Source: CAD feature listing. Evaluate the final solid. Frame: model axes, mm. Face numbers are marked on the shaded views. A direction names the side the tool comes from. Give positions to 0.01 mm unless a question says otherwise; leave off trailing zeros. Write each loop counter-clockwise with the first axis right and the second up, starting at its lowest first coordinate (ties: lowest second). Pieces come first, ordered by that corner, then holes. Notation, with made-up numbers: (27, 42) -> (46, 42) arc R21 cw to (46, 51) -> close; hole circle Ø4 at (63.25, 42.5). An arc over 180 degrees is marked (long way). Write item = value, one per line.
from build123d import *

# Parameters (mm, degrees)
SKETCH3_W           = 14.2875
SKETCH3_H           = 19.05
BOSS_EXTRUDE1_DEPTH = 22.225
SKETCH4_W           = 9.525
SKETCH4_H           = 7.9375
BOSS_EXTRUDE2_DEPTH = 6.35
SKETCH5_W           = 6.35
SKETCH5_H           = 19.05
CUT_EXTRUDE1_DEPTH  = 16.51


with BuildPart() as part:
    # Sketch3 → Boss-Extrude1 (new body)
    with BuildSketch(Plane(origin=(0, 0, 0), x_dir=(1, 0, 0), z_dir=(0, 1, 0))):
        Rectangle(SKETCH3_W, SKETCH3_H)
    extrude(amount=BOSS_EXTRUDE1_DEPTH)

    # Sketch4 → Boss-Extrude2 (add)
    with BuildSketch(Plane(origin=(0, 22.225, 0), x_dir=(1, 0, 0), z_dir=(0, 1, 0))):
        with Locations((0, 3.96875)):
            Rectangle(SKETCH4_W, SKETCH4_H)
    extrude(amount=BOSS_EXTRUDE2_DEPTH)

    # Sketch5 → Cut-Extrude1 (cut)
    with BuildSketch(Plane.XZ):
        Rectangle(SKETCH5_W, SKETCH5_H)
    extrude(amount=-CUT_EXTRUDE1_DEPTH, mode=Mode.SUBTRACT)


solid = part.part
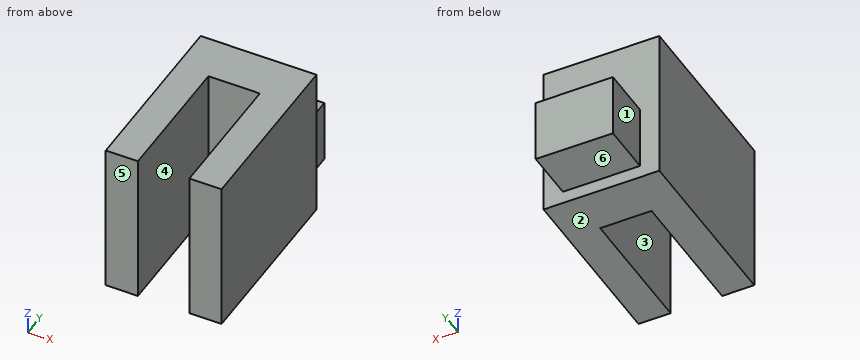
(1) Section query C-C (z = 8.25). Return loops of the section in (x, y) (3 decimals), plus the area to 3 significant figures.
Values follow:
outline = (-7.144, 0) -> (-3.175, 0) -> (-3.175, 16.51) -> (3.175, 16.51) -> (3.175, 0) -> (7.144, 0) -> (7.144, 22.225) -> (-7.144, 22.225) -> close
area = 213 mm2
(2) Access query for the marked faces 4, 5 and 6. Directions: +Z, -Z, +X, -X, +Y, -Y. A direction counts if a zero-diameter tool reaches every point of the face in a straight line with its end or side. Return the directions, or none.
Values follow:
face_4 = +Z, -Z, -Y
face_5 = +Z, -Z, +X, -X, -Y
face_6 = -Z, +X, -X, +Y
(3) Material intervals for line 1 (X direction, y = 5.25, z = 4.5) (3 decimals); line 2 (Y direction, x = 3.25, z = 1.75) (3 decimals); line 3 (X direction, y = 25.75, z = -6), sorted ascending.
Values follow:
line_1 = -7.144 to -3.175, 3.175 to 7.144
line_2 = 0 to 22.225
line_3 = -4.76 to 4.76
(4) Section query D-D (z = -5). Return loops of the section in (x, y) (1 decimal), plus the area to 3 significant figures.
Values follow:
outline = (-7.1, 0) -> (-3.2, 0) -> (-3.2, 16.5) -> (3.2, 16.5) -> (3.2, 0) -> (7.1, 0) -> (7.1, 22.2) -> (4.8, 22.2) -> (4.8, 28.6) -> (-4.8, 28.6) -> (-4.8, 22.2) -> (-7.1, 22.2) -> close
area = 273 mm2
(5) Section query B-B (x = 0.75). Return loops of the section in (y, z) (1 decimal), plus the area to 3 significant figures.
Values follow:
outline = (16.5, -9.5) -> (22.2, -9.5) -> (22.2, -7.9) -> (28.6, -7.9) -> (28.6, 0) -> (22.2, 0) -> (22.2, 9.5) -> (16.5, 9.5) -> close
area = 159 mm2
(6) Pull-direction query (X, two-part tool) for the marked faces 1, 2 and 3; classes: pulls with the +X half, pulls with the -X half, needs draft (parallel to the pull), parting line crosses it, or undercut.
Values follow:
face_1 = pulls with the -X half
face_2 = needs draft
face_3 = undercut
(7) Section query A-A (y = 12.75). Return loops of the section in (x, z) (3 decimals).
Values follow:
outline = (-7.144, -9.525) -> (-3.175, -9.525) -> (-3.175, 9.525) -> (-7.144, 9.525) -> close; (3.175, -9.525) -> (7.144, -9.525) -> (7.144, 9.525) -> (3.175, 9.525) -> close
(8) First-contact query: pin 1 (1.9 mm diameter, centred on x = -0.5, z = -3, fed in from -Y); pin 2 (3 mm diameter, centred on y = 26, z = -3, fed in from +X); pin 3 (7 mm diameter, centred on x = -2, y = 26.5, fed in from -Z); pin 4 (4 mm diameter, centred on x = 0, y = 8.5, fed in from +Z). Flat tips, straight axial feed; report the tip coordinate or a pass-through.
Values follow:
pin_1 = 16.51
pin_2 = 4.76
pin_3 = -7.94
pin_4 = through
